Geometry check sheet. Reference: drawing and pictorial views, mm from the part's lowest x, y, z. A direction names the side the tool comes from. Give positions to 0.01 mm unless a question says otherwise; leave off trailing zeros. Loops run counter-clockwise (first coordinate to the right, second up) from the corner with the lowest first, then second, coordinate; pieces in that order, holes last. Notation, with made-up numbers: (46.25, 2) - (95.25, 2) arc R17 cw to (95.25, 31) - close; hole circle Ø1 at (-31, -40). An arc over 180 degrees is marked (long way). Use CSV: the item, a comma, the result in double quotes.
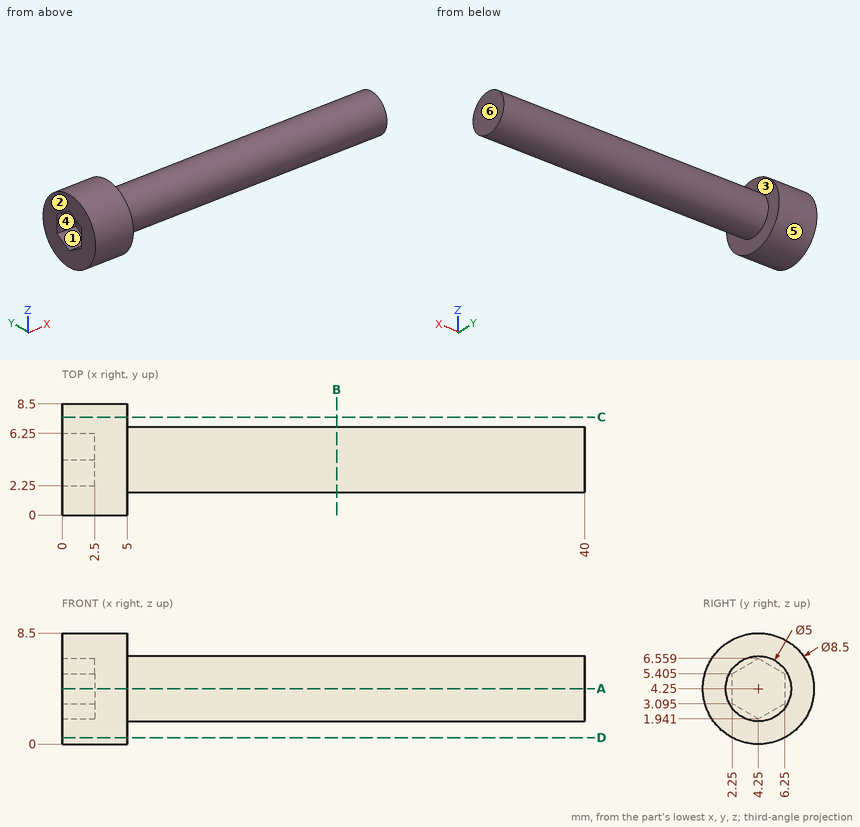
1. Set-up check for the marked faces 1, 2 and 3: record each of +Z, -Z, +X, -X, +Y, -Y from which the full face is reachable in a straight line by a thin tool's end or side.
Completed:
face 1,"-X"
face 2,"+Z, -Z, -X, +Y, -Y"
face 3,"+X"
2. Go/stop test with flat-tipped pins: pin 1 Ø2 at (x, y) = (19, 1) entering from +Z; pin 2 Ø1 at (x, y) = (30.5, 3) entering from +Z (1 decimal); pin 3 Ø2 at (x, z) = (13, 2.5) entering from -Y (1 decimal). Record where each tip stops, or that it passes through.
Completed:
pin 1,"stops at z = 5.34"
pin 2,"stops at z = 6.6"
pin 3,"stops at y = 1.9"
3. Sectioned sample at B-B, the plane x = 21. Record the boundary of the cut face in (y, z).
Completed:
outline,"circle Ø5 at (4.25, 4.25)"
4. Sectioned sample at D-D, the plane z = 0.5. Record the boundary of the cut face in (x, y), and give its area (3 significant figures).
Completed:
outline,"(0, 2.25) - (5, 2.25) - (5, 6.25) - (0, 6.25) - close"
area,"20.0 mm²"
5. Sectioned sample at C-C, the plane y = 7.5. Record the boundary of the cut face in (x, z).
Completed:
outline,"(0, 1.51) - (5, 1.51) - (5, 6.99) - (0, 6.99) - close"
6. Sectioned sample at A-A, the plane z = 4.25. Record the boundary of the cut face in (x, y).
Completed:
outline,"(0, 0) - (5, 0) - (5, 1.75) - (40, 1.75) - (40, 6.75) - (5, 6.75) - (5, 8.5) - (0, 8.5) - (0, 6.25) - (2.5, 6.25) - (2.5, 2.25) - (0, 2.25) - close"
7. Release check for a two-part mould opening along Y. For the marked faces 4, 5 and 6 record: released by +Y, released by -Y, zero draft, split by the parting line, or undercut.
Completed:
face 4,"undercut"
face 5,"split by the parting line"
face 6,"zero draft"
8. Scan lines: line 1 along X through (y, z) = (1.5, 1.75); line 2 along X through (y, z) = (4.75, 5); line 3 along Y through (x, z) = (30, 4.75). Record each from-to range of solid material in increasing order.
Completed:
line 1,"x = 0 to 5"
line 2,"x = 2.5 to 40"
line 3,"y = 1.8 to 6.7"
